Can you work these out from the model? Positions are in its coordinate system, mm. Face numbers are marked on the shaded views. Give positions to 0.01 mm unless a question says otherwise; leave off trailing zeros. Write each loop counter-clockwise with the first axis right and the second up, starting at its lowest first coordinate (ties: lowest second). Pieces come first, ordered by that corner, then holes. Notation, with made-up numbers: M 76,57 L 97,57 A9 cw 97,69 Z; hole C 27.25,-37.75 d3. An arc over 180 degrees is marked long. Write each question's results on one line, items separated by ' | '.
from build123d import *

# Parameters (mm, degrees)
SKETCH1_R           = 2.5
BOSS_EXTRUDE1_DEPTH = 100
FILLET1_R           = 1.065
FILLET2_R           = 2.13


with BuildPart() as part:
    # Sketch1 → Boss-Extrude1 (new body)
    with BuildSketch(Plane.YZ):
        Polygon((-12.5, -3.25), (-12.5, -12.5), (-3.25, -12.5), (-3.25, -10.37), (-8.863862556, -10.37), (-2.873862556, -4.38), (2.873862556, -4.38), (8.863862556, -10.37), (3.25, -10.37), (3.25, -12.5), (12.5, -12.5), (12.5, -3.25), (10.37, -3.25), (10.37, -8.863862556), (4.38, -2.873862556), (4.38, 2.873862556), (10.37, 8.863862556), (10.37, 3.25), (12.5, 3.25), (12.5, 12.5), (3.25, 12.5), (3.25, 10.37), (8.863862556, 10.37), (2.873862556, 4.38), (-2.873862556, 4.38), (-8.863862556, 10.37), (-3.25, 10.37), (-3.25, 12.5), (-12.5, 12.5), (-12.5, 3.25), (-10.37, 3.25), (-10.37, 8.863862556), (-4.38, 2.873862556), (-4.38, -2.873862556), (-10.37, -8.863862556), (-10.37, -3.25), align=None)
        with Locations(Location((0, 0, 0), (0, 0, 270))):
            Circle(SKETCH1_R, mode=Mode.SUBTRACT)
    extrude(amount=BOSS_EXTRUDE1_DEPTH)

    # Fillet1
    fillet1_edges = [part.edges().sort_by_distance(p)[0] for p in [
        (50, -10.37, -8.863862556),
        (50, 2.873862556, -4.38),
        (50, -2.873862556, -4.38),
        (50, -4.38, 2.873862556),
        (50, -4.38, -2.873862556),
        (50, -2.873862556, 4.38),
        (50, 2.873862556, 4.38),
        (50, 4.38, 2.873862556),
        (50, 4.38, -2.873862556),
        (50, -8.863862556, -10.37),
        (50, 8.863862556, -10.37),
        (50, 10.37, -8.863862556),
        (50, -10.37, 8.863862556),
        (50, -8.863862556, 10.37),
        (50, 10.37, 8.863862556),
        (50, 8.863862556, 10.37),
        (50, 12.5, 3.25),
        (50, -3.25, -12.5),
        (50, -10.37, 3.25),
        (50, 10.37, 3.25),
        (50, -10.37, -3.25),
        (50, -12.5, -3.25),
        (50, -12.5, 3.25),
        (50, 3.25, -10.37),
        (50, -3.25, -10.37),
        (50, 3.25, -12.5),
        (50, 10.37, -3.25),
        (50, 12.5, -3.25),
        (50, 3.25, 12.5),
        (50, 3.25, 10.37),
        (50, -3.25, 10.37),
        (50, -3.25, 12.5),
    ]]
    fillet(fillet1_edges, radius=FILLET1_R - 0.0001)  # a hair under: the kernel refuses the full size

    # Fillet2
    fillet2_edges = [part.edges().sort_by_distance(p)[0] for p in [
        (50, -12.5, 12.5),
        (50, 12.5, 12.5),
        (50, 12.5, -12.5),
        (50, -12.5, -12.5),
    ]]
    fillet(fillet2_edges, radius=FILLET2_R)


solid = part.part
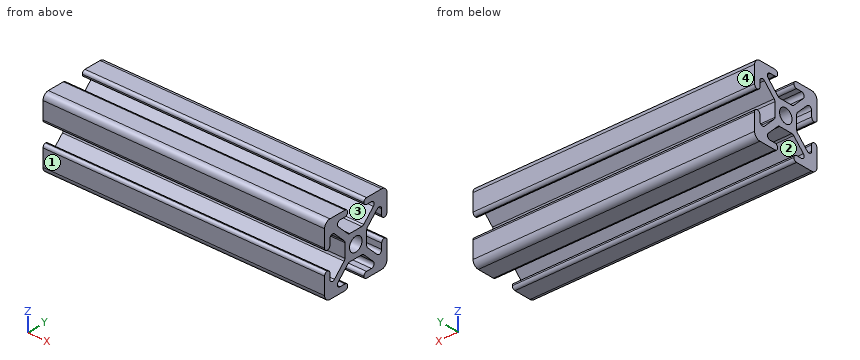
Item 1: Thinking about a two-plate mould opening in Y: for the marked faces 1, 2, 3 and 4, which applies, +Y half, -Y half, draft (parallel to the pull), parting line (faces both ways), or undercut?
Geometry says:
face 1: -Y half | face 2: undercut | face 3: undercut | face 4: +Y half
Item 2: If I drill on line 1 (Y direction, x = 50, z = 0); line 2 (Y direction, x = 11, z = -7.25); line 3 (Z direction, x = 83, y = -6.5), over which ranges is the centre line in solid material (lowest first)? Write a range as from..to.
Geometry says:
line 1: y = -4.38..-2.5, 2.5..4.38 | line 2: y = -12.5..-9.77, -8.84..-5.74, 5.74..8.84, 9.77..12.5 | line 3: z = -12.5..-10.35, -8.01..-4.99, 4.99..8.01, 10.35..12.5
Item 3: I want a section at A-A, the plane z = 0. Please give me the cut outline in (x, y), and give its area (3 significant figures).
Geometry says:
outline: M 0,-4.38 L 100,-4.38 L 100,-2.5 L 0,-2.5 Z; M 0,2.5 L 100,2.5 L 100,4.38 L 0,4.38 Z | area: 376 mm2
